The listing builds one solid part. Answer for the finished solid, in the listing's coordinates (mm). Give positions to 0.01 mm unless a question says otherwise; leave off trailing zeros. Write each loop counter-clockwise with the first axis right and the second up, starting at its lowest first coordinate (ties: lowest second). Pieces come first, ordered by that corner, then holes. Notation, with made-up numbers: M -27.75,-40 L 1.25,-40 A38 cw 1.25,-1 Z; hole C 66.25,31.25 d2. An arc over 180 degrees is marked long. Answer as a JSON object with one key per item and string values.
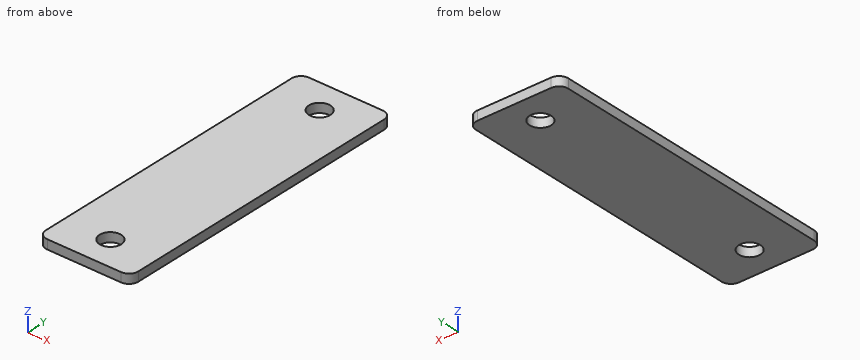
Autodesk Inventor part; units mm, degrees
ref_plane "YZ Plane" through (0, 0, 0) normal (1, 0, 0) x (0, 1, 0)
ref_plane "XZ Plane" through (0, 0, 0) normal (0, 1, 0) x (-1, 0, 0)
ref_plane "XY Plane" through (0, 0, 0) normal (0, 0, 1) x (1, 0, 0)
sketch "Sketch1" plane through (0, 0, 0) normal (0, 0, 1) x (1, 0, 0)
  line L0 (-30, -100) -> (30, -100)
  line L1 (30, -100) -> (30, 100)
  line L2 (30, 100) -> (-30, 100)
  line L3 (-30, 100) -> (-30, -100)
  line L4 (-30, -100) -> (30, 100) construction
  line L5 (30, -100) -> (-30, 100) construction
  circle A0 centre (0, 80) radius 7
  circle A1 centre (0, -80) radius 7
  line L6 (0, 100) -> (0, -100) construction
  line L7 (-30, 0) -> (30, 0) construction
  point P0 (0, 0)
  point P1 (0, 0)
  dimension "d154" = 60
  dimension "d155" = 200
  dimension "d157" = 20
  dimension "d159" = 14
extrude "Plate5" add sketch "Sketch1" along normal blind 6
fillet "Corner Round1" radius 6 4 edges at (-30, 100, 3) (30, 100, 3) (30, -100, 3) (-30, -100, 3)
1. A cutting plane is placed at A-A, the plane z = 4.7. Give the vertices of the cut face in (x, y).
Verdict:
{"outline": "M -30,-94 A6 ccw -24,-100 L 24,-100 A6 ccw 30,-94 L 30,94 A6 ccw 24,100 L -24,100 A6 ccw -30,94 Z; hole C 0,-80 d14; hole C 0,80 d14"}
2. A cutting plane is placed at B-B, the plane y = 80. Give the vertices of the cut face in (x, z), plus the area to 3 significant figures.
Verdict:
{"outline": "M -30,0 L -7,0 L -7,6 L -30,6 Z; M 7,0 L 30,0 L 30,6 L 7,6 Z", "area": "276 mm2"}
3. A cutting plane is placed at C-C, the plane x = 0. Give the vertices of the cut face in (y, z).
Verdict:
{"outline": "M -100,0 L -87,0 L -87,6 L -100,6 Z; M -73,0 L 73,0 L 73,6 L -73,6 Z; M 87,0 L 100,0 L 100,6 L 87,6 Z"}
4. Consider line 1 along Y through (x, z) = (0, 2.35); line 2 along Y through (x, z) = (-3, 5.75); line 3 along X through (y, z) = (78, 2.75). Determine where each line is inside the solid, lowest interval first.
Verdict:
{"line 1": "y = -100 to -87, -73 to 73, 87 to 100", "line 2": "y = -100 to -86.32, -73.68 to 73.68, 86.32 to 100", "line 3": "x = -30 to -6.71, 6.71 to 30"}
